Read the model definition and answer for the solid it produces. Units are mm, in the model's axes. A direction names the side the tool comes from. Coordinates: 2 decimals unless noted, no trailing zeros. Order: outer loops, then holes, each group sorted by start corner. A loop starts at its lowest first (then second) coordinate and runs counter-clockwise, first axis right, second up. Notation, with made-up numbers: (-33, -31.75) -> (-3, -31.75) arc R16 cw to (-3, -4.75) -> close; hole circle Ø3 at (72.25, 40). An arc over 180 degrees is marked (long way). Return JSON: item names as keys, results as strings. Group by question number.
Solid Edge part; units mm, degrees
sketch "Sketch1" plane through (0, 0, 0) normal (0, -1, 0) x (1, 0, 0)
  circle A0 centre (-47.8251, 6.7192) radius 60
extrude "Protrusion1" add sketch "Sketch1" against normal blind 200
sketch "Sketch2" plane through (-47.8251, 0, 6.7192) normal (0, -1, 0) x (1, 0, 0)
  circle A0 centre (0, 0) radius 5
extrude "ExtrudedProtrusion_3" add sketch "Sketch2" along normal blind 10
sketch "Sketch3" plane through (-47.8251, 200, 6.7192) normal (0, 1, 0) x (-1, 0, 0)
  circle A0 centre (0, 0) radius 5
extrude "ExtrudedProtrusion_4" add sketch "Sketch3" along normal blind 10
1. Straight lines are drawn through the part: L1, parallel to X at y = 61, z = 6.5; L2, parallel to Y at x = -26.5, z = -17.5; L3, parallel to X at y = 173.5, z = 9. For each, find the intervals that lie inside material, in ascending order.
2. Which of the six approach directions +Z, -Z, +X, -X, +Y, -Y give full straight-line access (tool end or side, diameter ignored) to faces 1 (the face through (-48, 210, 7)), 2 (the face through (-43.056, -4.93, 5.217)), 3 (the face through (-42.83, 204.93, 6.5))?
3. Find section A-A on z = 37. Determine the outline of the cut face in (x, y).
4. Find section B-B on x = -75.5. Determine the outline of the cut face in (y, z).
5. Given pin 1 (6 mm diameter, centred on y = 182, z = -11, fed in from -X); pin 2 (8 mm diameter, centred on x = -50, y = 70, fed in from +Z); pin 3 (1.5 mm diameter, centred on x = -14, z = 53, fed in from -Y), each flat-ended and moving along its own axis, determine where each tip first touches the part or whether it passes through.
6. Find section C-C on y = 117. Determine the outline of the cut face in (x, z).
Result:
{
 "1": {"L1": "-107.82 to 12.17", "L2": "0 to 200", "L3": "-107.78 to 12.13"},
 "2": {"face 1": "+Z, -Z, +X, -X, +Y", "face 2": "-Y", "face 3": "+Y"},
 "3": {"outline": "(-99.62, 0) -> (3.97, 0) -> (3.97, 200) -> (-99.62, 200) -> close"},
 "4": {"outline": "(0, -46.52) -> (200, -46.52) -> (200, 59.96) -> (0, 59.96) -> close"},
 "5": {"pin 1": "x = -105.99", "pin 2": "z = 66.72", "pin 3": "y = 0"},
 "6": {"outline": "circle Ø120 at (-47.83, 6.72)"}
}
